Could you check a few things on this model? Use its own coordinates, in mm. A direction names the side the tool comes from. Give positions to 0.01 mm unless a question says otherwise; leave off trailing zeros. Order: outer loops, then holes, each group sorted by start corner. A loop starts at its lowest first (then second) coordinate and runs counter-clockwise, first axis right, second up.
from build123d import *

# Parameters (mm, degrees)
ESQUISSE1_W                      = 440
ESQUISSE1_H                      = 220
BOSS_EXTRU_1_DEPTH               = 3
ESQUISSE2_R                      = 16
ENL_V_MAT_TUBE_DEPTH             = 3
ESQUISSE4_W                      = 20
ESQUISSE4_H                      = 3
ENL_V_MAT_C_T_ARRI_REBOITE_DEPTH = 3
ESQUISSE5_W                      = 3
ESQUISSE5_H                      = 20
ENL_V_MAT_C_T_DGBOITE_DEPTH      = 3
ENL_V_MAT_EXTRU_1_DEPTH          = 3


with BuildPart() as part:
    # Esquisse1 → Boss.-Extru.1 (new body)
    with BuildSketch(Plane.XY):
        Rectangle(ESQUISSE1_W, ESQUISSE1_H)
    extrude(amount=BOSS_EXTRU_1_DEPTH)

    # Esquisse2 → Enlèv. mat._Tube (cut)
    with BuildSketch(Plane(origin=(0, 0, 0), x_dir=(-1, 0, 0), z_dir=(0, 0, -1))):
        with Locations((-185, 78)):
            Circle(ESQUISSE2_R)
        with Locations((185, 78)):
            Circle(ESQUISSE2_R)
        with Locations((0, -65)):
            Circle(ESQUISSE2_R)
    extrude(amount=-ENL_V_MAT_TUBE_DEPTH, mode=Mode.SUBTRACT)

    # Esquisse4 → Enlèv. mat._CôtéArrièreBoite (cut)
    with BuildSketch(Plane(origin=(0, 0, 0), x_dir=(-1, 0, 0), z_dir=(0, 0, -1))):
        with Locations((-195, 105.5)):
            Rectangle(ESQUISSE4_W, ESQUISSE4_H)
        with Locations((-165, 105.5)):
            Rectangle(ESQUISSE4_W, ESQUISSE4_H)
        with Locations((-135, 105.5)):
            Rectangle(ESQUISSE4_W, ESQUISSE4_H)
        with Locations((-105, 105.5)):
            Rectangle(ESQUISSE4_W, ESQUISSE4_H)
        with Locations((-75, 105.5)):
            Rectangle(ESQUISSE4_W, ESQUISSE4_H)
        with Locations((-45, 105.5)):
            Rectangle(ESQUISSE4_W, ESQUISSE4_H)
        with Locations((-15, 105.5)):
            Rectangle(ESQUISSE4_W, ESQUISSE4_H)
        with Locations((15, 105.5)):
            Rectangle(ESQUISSE4_W, ESQUISSE4_H)
        with Locations((45, 105.5)):
            Rectangle(ESQUISSE4_W, ESQUISSE4_H)
        with Locations((75, 105.5)):
            Rectangle(ESQUISSE4_W, ESQUISSE4_H)
        with Locations((105, 105.5)):
            Rectangle(ESQUISSE4_W, ESQUISSE4_H)
        with Locations((135, 105.5)):
            Rectangle(ESQUISSE4_W, ESQUISSE4_H)
        with Locations((165, 105.5)):
            Rectangle(ESQUISSE4_W, ESQUISSE4_H)
        with Locations((195, 105.5)):
            Rectangle(ESQUISSE4_W, ESQUISSE4_H)
        with Locations((105, -105.5)):
            Rectangle(ESQUISSE4_W, ESQUISSE4_H)
        with Locations((135, -105.5)):
            Rectangle(ESQUISSE4_W, ESQUISSE4_H)
        with Locations((165, -105.5)):
            Rectangle(ESQUISSE4_W, ESQUISSE4_H)
        with Locations((195, -105.5)):
            Rectangle(ESQUISSE4_W, ESQUISSE4_H)
        with Locations((75, -105.5)):
            Rectangle(ESQUISSE4_W, ESQUISSE4_H)
        with Locations((45, -105.5)):
            Rectangle(ESQUISSE4_W, ESQUISSE4_H)
        with Locations((15, -105.5)):
            Rectangle(ESQUISSE4_W, ESQUISSE4_H)
        with Locations((-15, -105.5)):
            Rectangle(ESQUISSE4_W, ESQUISSE4_H)
        with Locations((-45, -105.5)):
            Rectangle(ESQUISSE4_W, ESQUISSE4_H)
        with Locations((-75, -105.5)):
            Rectangle(ESQUISSE4_W, ESQUISSE4_H)
        with Locations((-105, -105.5)):
            Rectangle(ESQUISSE4_W, ESQUISSE4_H)
        with Locations((-135, -105.5)):
            Rectangle(ESQUISSE4_W, ESQUISSE4_H)
        with Locations((-165, -105.5)):
            Rectangle(ESQUISSE4_W, ESQUISSE4_H)
        with Locations((-195, -105.5)):
            Rectangle(ESQUISSE4_W, ESQUISSE4_H)
    extrude(amount=-ENL_V_MAT_C_T_ARRI_REBOITE_DEPTH, mode=Mode.SUBTRACT)

    # Esquisse5 → Enlèv. mat.-CôtéDGBoite (cut)
    with BuildSketch(Plane(origin=(0, 0, 0), x_dir=(-1, 0, 0), z_dir=(0, 0, -1))):
        with Locations((-215.5, -90)):
            Rectangle(ESQUISSE5_W, ESQUISSE5_H)
        with Locations((-215.5, -60)):
            Rectangle(ESQUISSE5_W, ESQUISSE5_H)
        with Locations((-215.5, -30)):
            Rectangle(ESQUISSE5_W, ESQUISSE5_H)
        with Locations((-215.5, 0)):
            Rectangle(ESQUISSE5_W, ESQUISSE5_H)
        with Locations((-215.5, 30)):
            Rectangle(ESQUISSE5_W, ESQUISSE5_H)
        with Locations((-215.5, 60)):
            Rectangle(ESQUISSE5_W, ESQUISSE5_H)
        with Locations((-215.5, 90)):
            Rectangle(ESQUISSE5_W, ESQUISSE5_H)
        with Locations((215.5, 90)):
            Rectangle(ESQUISSE5_W, ESQUISSE5_H)
        with Locations((215.5, 60)):
            Rectangle(ESQUISSE5_W, ESQUISSE5_H)
        with Locations((215.5, 30)):
            Rectangle(ESQUISSE5_W, ESQUISSE5_H)
        with Locations((215.5, 0)):
            Rectangle(ESQUISSE5_W, ESQUISSE5_H)
        with Locations((215.5, -30)):
            Rectangle(ESQUISSE5_W, ESQUISSE5_H)
        with Locations((215.5, -60)):
            Rectangle(ESQUISSE5_W, ESQUISSE5_H)
        with Locations((215.5, -90)):
            Rectangle(ESQUISSE5_W, ESQUISSE5_H)
    extrude(amount=-ENL_V_MAT_C_T_DGBOITE_DEPTH, mode=Mode.SUBTRACT)

    # Esquisse6 → Enlèv. mat.-Extru.1 (cut)
    with BuildSketch(Plane(origin=(0, 0, 0), x_dir=(-1, 0, 0), z_dir=(0, 0, -1))):
        Polygon((-170, 20), (-117.084973779, 80), (-35, 80), (-35, -20), (-87.915026221, -80), (-170, -80), align=None)
        Polygon((170, 20), (170, -80), (87.915026221, -80), (35, -20), (35, 80), (117.084973779, 80), align=None)
    extrude(amount=-ENL_V_MAT_EXTRU_1_DEPTH, mode=Mode.SUBTRACT)


solid = part.part
Item 1: Please list where these lines run through material, in increasing order: line 1 along X through (y, z) = (0.5, 1.95); line 2 along X through (y, z) = (12, 0.3); line 3 along Y through (x, z) = (20.5, 1.5).
Findings:
line 1: x = -220 to -217, -214 to -170, -35 to 35, 170 to 214, 217 to 220
line 2: x = -220 to -170, -35 to 35, 170 to 220
line 3: y = -110 to -107, -104 to 104, 107 to 110
Item 2: Imagine slicing it at D-D on z = 0.5. Give the number of separate pieces and of enclosed holes in the cut face, then the cut area to 3 significant figures.
Findings:
separate pieces: 1
enclosed holes: 47
area: 55,000 mm2
Item 3: We'd pull the mould along X, two halves only. Please class faces 3 (the flat face through (-61.83, -50.42, 1.48)), 4 (the flat face through (-3, 2, 0)), 5 (the flat face through (143.913, 49.58, 1.479)): +X half, -X half, draft (parallel to the pull), parting line (faces both ways), or undercut.
Findings:
face 3: undercut
face 4: draft
face 5: undercut
Item 4: Imagine slicing it at B-B on x = 0. List the corners of the cut face in (y, z) for me, then the cut area to 3 significant figures.
Findings:
outline: (-110, 0) - (-81, 0) - (-81, 3) - (-110, 3) - close; (-49, 0) - (110, 0) - (110, 3) - (-49, 3) - close
area: 564 mm2
Item 5: For faces 1 (the flat face through (-3, 2, 3)), 2 (the flat face through (61.087, -49.58, 1.479)), which set-ups out of +Z, -Z, +X, -X, +Y, -Y let a thin tool reach every point of the face, with its end or its side?
Findings:
face 1: +Z, +X, -X, +Y, -Y
face 2: +Z, -Z
Item 6: Imagine slicing it at A-A on y = -16. List the corners of the cut face in (x, z) for me.
Findings:
outline: (-220, 0) - (-170, 0) - (-170, 3) - (-220, 3) - close; (-35, 0) - (35, 0) - (35, 3) - (-35, 3) - close; (170, 0) - (220, 0) - (220, 3) - (170, 3) - close
Item 7: Imagine slicing it at C-C on y = -65. List the corners of the cut face in (x, z) for me.
Findings:
outline: (-220, 0) - (-217, 0) - (-217, 3) - (-220, 3) - close; (-214, 0) - (-170, 0) - (-170, 3) - (-214, 3) - close; (-74.69, 0) - (-16, 0) - (-16, 3) - (-74.69, 3) - close; (16, 0) - (74.69, 0) - (74.69, 3) - (16, 3) - close; (170, 0) - (214, 0) - (214, 3) - (170, 3) - close; (217, 0) - (220, 0) - (220, 3) - (217, 3) - close
